from build123d import *

# Parameters (mm, degrees)
F0_W     = 24.8156127766
F0_H     = 70
F1_DEPTH = 17.79
F0_R     = 7.5
F2_DEPTH = 8.085
F3_DEPTH = 8.085


with BuildPart() as f1:
    # F0 (on Top) → F1 (new body)
    with BuildSketch(Plane.XY):
        with Locations((12.4078063883, 0)):
            Rectangle(F0_W, F0_H)
        with Locations((-12.4078063883, 0)):
            Rectangle(F0_W, F0_H)
    extrude(amount=F1_DEPTH)

    # F0 (on Top) → F2 (join)
    with BuildSketch(Plane.XY):
        with BuildLine():
            Line((24.8156127766, 35), (24.8156127766, -35))
            Line((24.8156127766, -35), (24.8156127766, -44.395))
            Line((24.8156127766, -44.395), (63.155, -44.395))
            ThreePointArc((63.155, -44.395), (66.6905339059, -42.9305339059), (68.155, -39.395))
            Line((68.155, -39.395), (68.155, 39.395))
            ThreePointArc((68.155, 39.395), (66.6905339059, 42.9305339059), (63.155, 44.395))
            Line((63.155, 44.395), (24.8156127766, 44.395))
            Line((24.8156127766, 44.395), (24.8156127766, 35))
        make_face()
        with Locations((47.5, -22.8035077453)):
            Circle(F0_R, mode=Mode.SUBTRACT)
        with Locations((47.5, 22.1964922547)):
            Circle(F0_R, mode=Mode.SUBTRACT)
        with BuildLine():
            Line((-24.8156127766, -44.395), (-24.8156127766, -35))
            Line((-24.8156127766, -35), (-24.8156127766, 35))
            Line((-24.8156127766, 35), (-24.8156127766, 44.395))
            Line((-24.8156127766, 44.395), (-63.155, 44.395))
            ThreePointArc((-63.155, 44.395), (-66.6905339059, 42.9305339059), (-68.155, 39.395))
            Line((-68.155, 39.395), (-68.155, -39.395))
            ThreePointArc((-68.155, -39.395), (-66.6905339059, -42.9305339059), (-63.155, -44.395))
            Line((-63.155, -44.395), (-24.8156127766, -44.395))
        make_face()
        with Locations((-47.5, -22.8035077453)):
            Circle(F0_R, mode=Mode.SUBTRACT)
        with Locations((-47.5, 22.1964922547)):
            Circle(F0_R, mode=Mode.SUBTRACT)
    extrude(amount=F2_DEPTH)

    # F0 (on Top) → F3 (join)
    with BuildSketch(Plane.XY):
        with BuildLine():
            Line((-24.8156127766, -44.395), (-24.8156127766, -35))
            Line((-24.8156127766, -35), (-24.8156127766, 35))
            Line((-24.8156127766, 35), (-24.8156127766, 44.395))
            Line((-24.8156127766, 44.395), (-63.155, 44.395))
            ThreePointArc((-63.155, 44.395), (-66.6905339059, 42.9305339059), (-68.155, 39.395))
            Line((-68.155, 39.395), (-68.155, -39.395))
            ThreePointArc((-68.155, -39.395), (-66.6905339059, -42.9305339059), (-63.155, -44.395))
            Line((-63.155, -44.395), (-24.8156127766, -44.395))
        make_face()
        with Locations((-47.5, -22.8035077453)):
            Circle(F0_R, mode=Mode.SUBTRACT)
        with Locations((-47.5, 22.1964922547)):
            Circle(F0_R, mode=Mode.SUBTRACT)
        with BuildLine():
            Line((24.8156127766, 35), (24.8156127766, -35))
            Line((24.8156127766, -35), (24.8156127766, -44.395))
            Line((24.8156127766, -44.395), (63.155, -44.395))
            ThreePointArc((63.155, -44.395), (66.6905339059, -42.9305339059), (68.155, -39.395))
            Line((68.155, -39.395), (68.155, 39.395))
            ThreePointArc((68.155, 39.395), (66.6905339059, 42.9305339059), (63.155, 44.395))
            Line((63.155, 44.395), (24.8156127766, 44.395))
            Line((24.8156127766, 44.395), (24.8156127766, 35))
        make_face()
        with Locations((47.5, -22.8035077453)):
            Circle(F0_R, mode=Mode.SUBTRACT)
        with Locations((47.5, 22.1964922547)):
            Circle(F0_R, mode=Mode.SUBTRACT)
    extrude(amount=-F3_DEPTH)


solid = f1.part
Design review of the part built by this model. Coordinates are the model's own, in mm. A direction names the side the tool comes from. Give positions to 0.01 mm unless a question says otherwise; leave off trailing zeros. Order: outer loops, then holes, each group sorted by start corner. A loop starts at its lowest first (then second) coordinate and runs counter-clockwise, first axis right, second up. Notation, with made-up numbers: (15, 67.25) - (57, 67.25) arc R13 ccw to (57, 90.25) - close; hole circle Ø4 at (-34.75, -28). An arc over 180 degrees is marked (long way). Write item = value, one per line. Start each with the question number.
Q1. We need section C-C on y = 38. State the section outline as (x, z) points (3 decimals).
Q2. Clearance check with flat-ended pins moving along their axes: pin 1 Ø12 at (x, y) = (-47.5, -22.8) entering from -Z; pin 2 Ø15 at (x, y) = (3.5, -11) entering from -Z; pin 3 Ø24 at (x, y) = (-47.5, 22.2) entering from +Z (3 decimals); pin 4 Ø1 at (x, z) = (-2, 3) entering from -Y. State where each tip first meets the part, or that it passes through.
Q3. Mouldability with a two-part tool opening along X and no side actions: class faces 1 (the face through (0, 0, 17.79)), 2 (the face through (0, -35, 9)), 3 (the face through (-24.816, 0, 13)), 4 (the face through (0, 35, 9)) as released by +X, released by -X, zero draft, split by the parting line, or undercut.
Q4. We need section D-D on y = -12.5. State the section outline as (x, z) points (3 decimals).
Q5. We need section A-A on z = -2. State the section outline as (x, y) points (1 decimal).
Q6. Tool access review of faces 5 (the face through (46, 1, 8.085)), 6 (the face through (0, 0, 0)), 7 (the face through (-47, 1, 8.085)), 8 (the face through (-66.65, 42.97, 0.11)): name each direction out of +Z, -Z, +X, -X, +Y, -Y from which nothing blocks a thin tool from reaching the whole face with its end or side.
Q7. We need section B-B on x = -47.5. State the section outline as (y, z) points (1 decimal), plus the area to 3 significant figures.
Q8. To check wall thickness, follow L1, parallel to Y at x = -47.5, z = 5 (1 decimal); L2, parallel to X at y = 18, z = -5.75 (3 decimals); L3, parallel to X at y = 25, z = -3 (3 decimals). State the ranges of each line that lie inside material, in increasing order. Write a range as from..to.
Working result:
q1.outline = (-68.155, -8.085) - (-24.816, -8.085) - (-24.816, 8.085) - (-68.155, 8.085) - close; (24.816, -8.085) - (68.155, -8.085) - (68.155, 8.085) - (24.816, 8.085) - close
q2.pin_1 = through
q2.pin_2 = 0
q2.pin_3 = 8.085
q2.pin_4 = -35
q3.face_1 = zero draft
q3.face_2 = undercut
q3.face_3 = released by -X
q3.face_4 = undercut
q4.outline = (-68.155, -8.085) - (-24.816, -8.085) - (-24.816, 0) - (24.816, 0) - (24.816, -8.085) - (68.155, -8.085) - (68.155, 8.085) - (24.816, 8.085) - (24.816, 17.79) - (-24.816, 17.79) - (-24.816, 8.085) - (-68.155, 8.085) - close
q5.outline = (-68.2, -39.4) arc R5 ccw to (-63.2, -44.4) - (-24.8, -44.4) - (-24.8, 44.4) - (-63.2, 44.4) arc R5 ccw to (-68.2, 39.4) - close; (24.8, -44.4) - (63.2, -44.4) arc R5 ccw to (68.2, -39.4) - (68.2, 39.4) arc R5 ccw to (63.2, 44.4) - (24.8, 44.4) - close; hole circle Ø15 at (-47.5, -22.8); hole circle Ø15 at (-47.5, 22.2); hole circle Ø15 at (47.5, -22.8); hole circle Ø15 at (47.5, 22.2)
q6.face_5 = +Z, +X, +Y, -Y
q6.face_6 = -Z, +Y, -Y
q6.face_7 = +Z, -X, +Y, -Y
q6.face_8 = +Z, -Z, -X, +Y
q7.outline = (-44.4, -8.1) - (-30.3, -8.1) - (-30.3, 8.1) - (-44.4, 8.1) - close; (-15.3, -8.1) - (14.7, -8.1) - (14.7, 8.1) - (-15.3, 8.1) - close; (29.7, -8.1) - (44.4, -8.1) - (44.4, 8.1) - (29.7, 8.1) - close
q7.area = 951 mm²
q8.L1 = -44.4..-30.3, -15.3..14.7, 29.7..44.4
q8.L2 = -68.155..-53.716, -41.284..-24.816, 24.816..41.284, 53.716..68.155
q8.L3 = -68.155..-54.456, -40.544..-24.816, 24.816..40.544, 54.456..68.155
